Could you check a few things on this model? Use its own coordinates, in mm. Face numbers are marked on the shaded views. Coordinates: 2 decimals unless noted, no trailing zeros. Loops run counter-clockwise (first coordinate to the right, second up) from the corner with the lowest first, then second, coordinate; pieces in that order, holes last. Notation, with made-up numbers: M 29.5,-1 L 64.5,-1 A18 cw 64.5,5 Z; hole C -38,-26 d1. An arc over 180 degrees is marked long. Return JSON: item names as keys, results as strings. Group by question number.
from build123d import *

# Parameters (mm, degrees)
SKETCH3_R                = 40.005
BOSS_EXTRUDE1_DEPTH      = 20.14
SKETCH4_R                = 38.1
CUT_EXTRUDE1_DEPTH       = 20.14
SKETCH2_R                = 49.03
BOSS_EXTRUDE2_DEPTH      = 1.05
SKETCH6_R                = 38.1
CUT_EXTRUDE2_DEPTH       = 1.05
M1_2X0_25_TAPPED_HOLE2_D = 0.95


with BuildPart() as part:
    # Sketch3 → Boss-Extrude1 (new body)
    with BuildSketch(Plane(origin=(0, 0, 0), x_dir=(1, 0, 0), z_dir=(0, 1, 0))):
        Circle(SKETCH3_R)
    extrude(amount=BOSS_EXTRUDE1_DEPTH)

    # Sketch4 → Cut-Extrude1 (cut)
    with BuildSketch(Plane(origin=(0, 20.14, 0), x_dir=(1, 0, 0), z_dir=(0, 1, 0))):
        Circle(SKETCH4_R)
    extrude(amount=-CUT_EXTRUDE1_DEPTH, mode=Mode.SUBTRACT)

    # Sketch2 → Boss-Extrude2 (add)
    with BuildSketch(Plane(origin=(0, 0, 0), x_dir=(1, 0, 0), z_dir=(0, 1, 0))):
        Circle(SKETCH2_R)
    extrude(amount=BOSS_EXTRUDE2_DEPTH)

    # Sketch6 → Cut-Extrude2 (cut)
    with BuildSketch(Plane(origin=(0, 1.05, 0), x_dir=(1, 0, 0), z_dir=(0, 1, 0))):
        Circle(SKETCH6_R)
    extrude(amount=-CUT_EXTRUDE2_DEPTH, mode=Mode.SUBTRACT)

    # M1.2x0.25 Tapped Hole2 (through all)
    with Locations(Plane(origin=(-12.298859085, 1.05, -44.559581921), x_dir=(0, 0, 1), z_dir=(0, 1, 0))):
        with Locations((0, 0), (-0.179575061, 23.927525232), (11.62866746, 44.739161663), (32.260724597, 56.858437128), (56.188247767, 57.038018412), (76.999884487, 45.229773054), (89.119161163, 24.597717695), (89.298738325, 0.670192913), (77.49049699, -20.141443547), (56.858440891, -32.260723471), (32.930915763, -32.440301841), (12.119282142, -20.63205416)):
            Hole(M1_2X0_25_TAPPED_HOLE2_D / 2)


solid = part.part
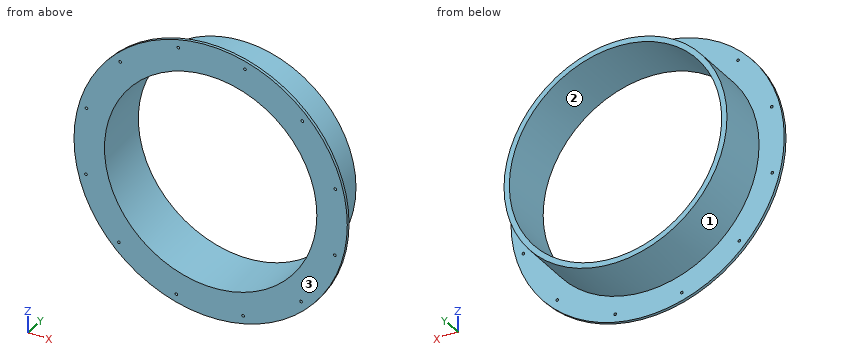
(1) Will these pins go through, and if not, where does the flat tip stop? P1, Ø4, axis at y = 15.5, z = 31, coming from the -X side; P2, Ø2, axis at x = 26, y = 9, coming from the +Z side; P3, Ø6, axis at x = 34.5, y = 12, coming from the +Z side; P4, Ø1.5, axis at x = -38.5, z = -1, coming from the -Y side.
(2) We'd pull the mould along Z, two halves only. Please class the marked faces 1, 2 and 3: +Z half, -Z half, draft (parallel to the pull), parting line (faces both ways), or undercut.
(3) Imagine slicing it at B-B, the plane x = 0. Write out the boundary of the cut face in (y, z) (3 decimals), then the cut area to 3 significant figures.
(4) If I drill on L1, parallel to X at y = 9, z = 0 (3 decimals); L2, parallel to Y at x = 19.5, z = -40, over which ranges is the centre line in solid material (lowest first)? Write a range as [from, to].
(5) Imagine slicing it at C-C, the plane y = 18.75. Write out the boundary of the cut face in (x, z) (3 decimals), then the cut area to 3 significant figures.
(6) Imagine slicing it at A-A, the plane z = 0. Write out the boundary of the cut face in (x, y) (3 decimals).
Checks:
{
 "1": {"P1": "x = -27.56", "P2": "z = 31.23", "P3": "z = 24.66", "P4": "y = 0"},
 "2": {"face 1": "parting line", "face 2": "undercut", "face 3": "draft"},
 "3": {"outline": "M 0,-49.03 L 1.05,-49.03 L 1.05,-40.005 L 20.14,-40.005 L 20.14,-38.1 L 0,-38.1 Z; M 0,38.1 L 20.14,38.1 L 20.14,40.005 L 1.05,40.005 L 1.05,49.03 L 0,49.03 Z", "area": "95.7 mm²"},
 "4": {"L1": "[-40.005, -38.1], [38.1, 40.005]", "L2": "[0, 1.05]"},
 "5": {"outline": "C 0,0 d80.01; hole C 0,0 d76.2", "area": "467 mm²"},
 "6": {"outline": "M -49.03,0 L -38.1,0 L -38.1,20.14 L -40.005,20.14 L -40.005,1.05 L -49.03,1.05 Z; M 38.1,0 L 49.03,0 L 49.03,1.05 L 40.005,1.05 L 40.005,20.14 L 38.1,20.14 Z"}
}
